Could you check a few things on this model? Use its own coordinates, in mm. Round coordinates to 2 decimals unless told otherwise and drop trailing zeros. Loops run counter-clockwise (first coordinate to the right, second up) from the corner with the lowest first, then second, coordinate; pieces in that order, holes last. Notation, with made-up numbers: (86.25, -38) -> (135.25, -38) arc R13 ccw to (135.25, -27) -> close; hole circle Ø4 at (46, 80). An arc over 180 degrees is marked (long way). One line per item, written item: value.
```python
from build123d import *


with BuildPart() as part:
    # Sketch1 → Revolve1 (revolve)
    with BuildSketch(Plane.XY, mode=Mode.PRIVATE) as revolve1_sk:
        with BuildLine():
            Line((0, 0), (24.360145845, 0))
            ThreePointArc((24.360145845, 0), (35.651483834, 4.677025332), (40.328509165, 15.96836332))
            Line((40.328509165, 15.96836332), (40.328509165, 67.23016629))
            ThreePointArc((40.328509165, 67.23016629), (38.415383352, 73.392914659), (33.348649325, 77.388878138))
            ThreePointArc((33.348649325, 77.388878138), (26.276782154, 81.308753559), (20.55607493, 87.022792188))
            Line((20.55607493, 87.022792188), (20.55607493, 96.024974169))
            Line((20.55607493, 96.024974169), (24.360145845, 96.024974169))
            Line((24.360145845, 96.024974169), (24.360145845, 98.393969428))
            Line((24.360145845, 98.393969428), (0, 98.393969428))
            Line((0, 98.393969428), (0, 0))
        make_face()
    revolve(revolve1_sk.sketch.rotate(Axis((0, 98.393969428, 0), (0, -1, 0)), 90), axis=Axis((0, 98.393969428, 0), (0, -1, 0)))


solid = part.part
```
Item 1: If we section it at B-B on z = 0: List the corners of the cut face in (x, y) for me.
Output:
outline: (-40.33, 15.97) arc R15.97 ccw to (-24.36, 0) -> (24.36, 0) arc R15.97 ccw to (40.33, 15.97) -> (40.33, 67.23) arc R10.88 ccw to (33.35, 77.39) arc R29.11 cw to (20.56, 87.02) -> (20.56, 96.02) -> (24.36, 96.02) -> (24.36, 98.39) -> (-24.36, 98.39) -> (-24.36, 96.02) -> (-20.56, 96.02) -> (-20.56, 87.02) arc R29.11 cw to (-33.35, 77.39) arc R10.88 ccw to (-40.33, 67.23) -> close
Item 2: If we section it at D-D on y = 82: List the corners of the cut face in (x, z) for me, plus the area to 3 significant figures.
Output:
outline: circle Ø50.79 at (0, 0)
area: 2,030 mm²
Item 3: Will these pins go through, and if not, where does the flat tip stop? pin 1 Ø12 at (x, y) = (15, 12.5) entering from -Z; pin 2 Ø12 at (y, z) = (21.5, 5.5) entering from -X; pin 3 Ø10 at (y, z) = (49.5, 23.5) entering from +X.
Output:
pin 1: stops at z = -39.16
pin 2: stops at x = -40.33
pin 3: stops at x = 35.83
Item 4: I need wall thicknesses on line 1 (Z direction, x = 0.5, y = 58.5); line 2 (X direction, y = 59, z = -26.5); line 3 (X direction, y = 54.5, z = -15). Which ranges of each line are inside material? Lowest first, please. Write a range as from..to.
Output:
line 1: z = -40.33..40.33
line 2: x = -30.4..30.4
line 3: x = -37.44..37.44
Item 5: If we section it at C-C on y = 52.5: List the corners of the cut face in (x, z) for me, plus the area to 3 significant figures.
Output:
outline: circle Ø80.66 at (0, 0)
area: 5,110 mm²
Item 6: If we section it at A-A on x = 0: List the corners of the cut face in (y, z) for me.
Output:
outline: (0, -24.36) arc R15.97 ccw to (15.97, -40.33) -> (67.23, -40.33) arc R10.88 ccw to (77.39, -33.35) arc R29.11 cw to (87.02, -20.56) -> (96.02, -20.56) -> (96.02, -24.36) -> (98.39, -24.36) -> (98.39, 24.36) -> (96.02, 24.36) -> (96.02, 20.56) -> (87.02, 20.56) arc R29.11 cw to (77.39, 33.35) arc R10.88 ccw to (67.23, 40.33) -> (15.97, 40.33) arc R15.97 ccw to (0, 24.36) -> close
Item 7: If we mould it in two halves opening along Y, with no side actions, what happens to faces 1 (the face through (-0.904, 91.587, -20.536)), 2 (the face through (18, 96.025, 11)), 3 (the face through (23.78, 97.23, -5.28)), 4 (the face through (0, 98.394, 0))? For each: released by +Y, released by -Y, zero draft, split by the parting line, or undercut.
Output:
face 1: undercut
face 2: undercut
face 3: zero draft
face 4: released by +Y
